The listing builds one solid part. Answer for the finished solid, in the listing's coordinates (mm). Face numbers are marked on the shaded views. Give positions to 0.01 mm unless a question says otherwise; leave off trailing zeros. Order: outer loops, then holes, each group sorted by start corner. A loop starts at its lowest first (then second) coordinate and runs counter-clockwise, first axis right, second up. Notation, with made-up numbers: (37, 58.25) -> (61, 58.25) arc R13 ccw to (61, 82.25) -> close; hole circle Ø4 at (22, 21.25). An arc over 180 degrees is marked (long way). Write item = value, one per line. Start each with the question number.
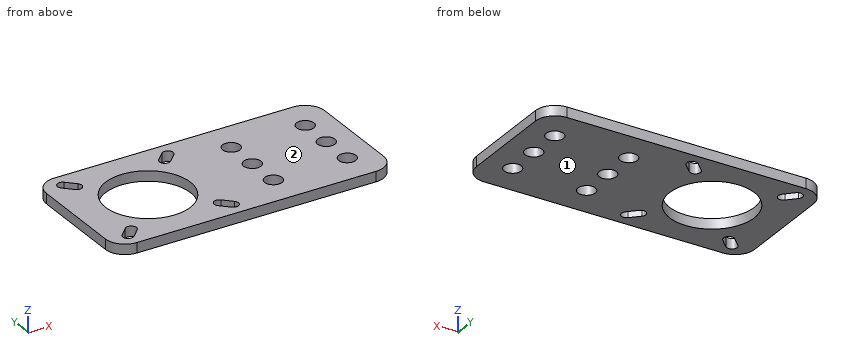
Autodesk Inventor part; units mm, degrees
ref_plane "Work Plane1" through (-41, 0, 0) normal (0, 1, 0) x (1, 0, 0)
ref_plane "Work Plane2" through (-19.75, 0, 3) normal (-1, 0, 0) x (0, 0, 1)
ref_plane "YZ Plane" through (0, 0, 0) normal (1, 0, 0) x (0, 1, 0)
sketch "Sketch1" plane through (0, 0, 0) normal (0, 0, 1) x (1, 0, 0)
  line L0 (-41, -19.75) -> (41, -19.75)
  line L1 (41, -19.75) -> (41, 19.75)
  line L2 (41, 19.75) -> (-41, 19.75)
  line L3 (-41, 19.75) -> (-41, -19.75)
  line L4 (-41, -19.75) -> (41, 19.75) construction
  line L5 (41, -19.75) -> (-41, 19.75) construction
  point P0 (0, 0)
  dimension "d0" = 82
  dimension "d1" = 39.5
extrude "Extrusion1" add sketch "Sketch1" along normal blind 3
sketch "Sketch2" plane through (0, 0, 3) normal (0, 0, 1) x (1, 0, 0)
  line L0 (-41, -19.75) -> (41, -19.75)
  line L1 (41, -19.75) -> (41, 19.75)
  line L2 (41, 19.75) -> (-41, 19.75)
  line L3 (-41, 19.75) -> (-41, -19.75)
  line L4 (-41, 0) -> (41, 0) construction
  line L5 (-19.75, 19.75) -> (-19.75, -19.75) construction
  point P0 (0, 0)
  point P1 (-19.75, 0)
  dimension "d4" = 21.25
hole "Hole1" at (-19.75, 0, 3) direction (0, 0, -1) diameter 25 end through all
sketch "Sketch3" plane through (0, 0, 3) normal (0, 0, 1) x (1, 0, 0)
  circle A0 centre (-19.75, 0) radius 12.5
  line L0 (-41, -19.75) -> (41, -19.75)
  line L1 (41, 19.75) -> (-41, 19.75)
  line L2 (-41, 19.75) -> (-41, -19.75)
  line L3 (-19.75, 0) -> (8.1807, 0) construction
  line L4 (-19.75, 0) -> (0, 19.75) construction
  line L5 (-19.75, 0) -> (8.1807, 0) construction
  line L6 (-19.75, 0) -> (0, -19.75) construction
  line L7 (-19.75, 0) -> (-39.5, 19.75) construction
  line L8 (-19.75, 0) -> (-39.5, -19.75) construction
  arc A1 (-31.654, -14.096) -> (-33.846, -11.904) centre (-32.75, -13) ccw
  arc A2 (-36.346, -14.404) -> (-34.154, -16.596) centre (-35.25, -15.5) ccw
  line L9 (-33.846, -11.904) -> (-36.346, -14.404)
  line L10 (-34.154, -16.596) -> (-31.654, -14.096)
  point P0 (0, 0)
  dimension "d13" = 45
  dimension "d14" = 5.75
  dimension "d15" = 8.25
  dimension "d16" = 35.25
  dimension "d17" = 32.75
  dimension "d18" = 3.1
  dimension "d19" = 3.1
extrude "Extrusion2" cut sketch "Sketch3" against normal through all contours L10 A2 L9 A1
ref_plane "Work Plane1" through (-41, 0, 0) normal (0, 1, 0) x (1, 0, 0)
ref_plane "Work Plane2" through (-19.75, 0, 3) normal (-1, 0, 0) x (0, 0, 1)
mirror "Mirror1" about plane through (-19.75, 0, 3) normal (-1, 0, 0) of "Extrusion2"
mirror "Mirror2" about plane through (-41, 0, 0) normal (0, 1, 0) of "Extrusion2", "Mirror1"
sketch "Sketch4" plane through (0, 0, 3) normal (0, 0, 1) x (1, 0, 0)
  circle A0 centre (-19.75, 0) radius 12.5
  line L0 (-41, -19.75) -> (41, -19.75)
  line L1 (41, -19.75) -> (41, 19.75)
  line L2 (41, 19.75) -> (-41, 19.75)
  line L3 (-41, 19.75) -> (-41, -19.75)
  line L4 (11, 19.75) -> (11, -19.75) construction
  line L5 (21.9, 19.75) -> (21.9, -19.75) construction
  line L6 (41, 0) -> (-41, 0) construction
  point P0 (0, 0)
  point P1 (11, 0)
  point P2 (11, 10)
  point P3 (11, -10)
  point P4 (32.8, 0)
  point P5 (32.8, 10)
  point P6 (32.8, -10)
  dimension "d22" = 52
  dimension "d23" = 10.9
  dimension "d24" = 10
  dimension "d25" = 8.2
  dimension "d26" = 9.75
  dimension "d27" = 21.8
  dimension "d28" = 30.75
hole "Hole2" at (11, 0, 3) at (11, 10, 3) at (11, -10, 3) at (32.8, -10, 3) at (32.8, 10, 3) at (32.8, 0, 3) direction (0, 0, -1) diameter 5.1 end through all
fillet "Fillet1" radius 5.75 4 edges at (-41, 19.75, 1.5) (-41, -19.75, 1.5) (41, -19.75, 1.5) (41, 19.75, 1.5)
equation "\"d19\" = d18"
properties part number "V-Slot Motor Mount Plate" material "Aluminum 6061"
Item 1: A cutting plane is placed at B-B, the plane y = 0. Write down the section's boundary in (x, z), plus the area to 3 significant figures.
Item 2: A cutting plane is placed at D-D, the plane y = -6. Write down the section's boundary in (x, z), plus the area to 3 significant figures.
Item 3: A cutting plane is placed at C-C, the plane z = 1.65. Count the separate pieces of the cut face and the enclosed holes in it, plus the area to 3 significant figures.
Item 4: A cutting plane is placed at A-A, the plane x = -19.75. Write down the section's boundary in (y, z).
Item 5: Consider L1, parallel to Y at x = 32.8, z = 1.2; L2, parallel to X at y = 0, z = 0.7; L3, parallel to Y at x = -5, z = 1.1. Determine where each line is inside the solid, lowest interval first. Write a range as from..to.
Item 6: The mould has two halves that part along Z. Classify the marked faces 1 and 2: +Z half, -Z half, draft (parallel to the pull), parting line (faces both ways), or undercut.
Check values:
q1.outline = (-41, 0) -> (-32.25, 0) -> (-32.25, 3) -> (-41, 3) -> close; (-7.25, 0) -> (8.45, 0) -> (8.45, 3) -> (-7.25, 3) -> close; (13.55, 0) -> (30.25, 0) -> (30.25, 3) -> (13.55, 3) -> close; (35.35, 0) -> (41, 0) -> (41, 3) -> (35.35, 3) -> close
q1.area = 140 mm^2
q2.outline = (-41, 0) -> (-30.72, 0) -> (-30.72, 3) -> (-41, 3) -> close; (-8.78, 0) -> (41, 0) -> (41, 3) -> (-8.78, 3) -> close
q2.area = 180 mm^2
q3.separate_pieces = 1
q3.enclosed_holes = 11
q3.area = 2,520 mm^2
q4.outline = (-19.75, 0) -> (-12.5, 0) -> (-12.5, 3) -> (-19.75, 3) -> close; (12.5, 0) -> (19.75, 0) -> (19.75, 3) -> (12.5, 3) -> close
q5.L1 = -19.75..-12.55, -7.45..-2.55, 2.55..7.45, 12.55..19.75
q5.L2 = -41..-32.25, -7.25..8.45, 13.55..30.25, 35.35..41
q5.L3 = -19.75..-16.86, -12.56..12.56, 16.86..19.75
q6.face_1 = -Z half
q6.face_2 = +Z half
